Read the model definition and answer for the solid it produces. Units are mm, in the model's axes. A direction names the side the tool comes from. Round coordinates to 2 decimals unless told otherwise and drop trailing zeros. Write each loop counter-clockwise with the first axis right and the second up, starting at its lowest first coordinate (ties: lowest second). Pieces come first, ordered by that corner, then holes. Notation, with made-up numbers: M -29.75,-4.5 L -3.75,-4.5 A20 ccw -3.75,6.5 Z; hole C 80,-27.75 d11. An arc over 180 degrees is marked long. Use one line per item in the form item = value. Start each with the question number.
```python
from build123d import *

# Parameters (mm, degrees)
SKETCH3_W               = 6.6929
SKETCH3_H               = 0.635
CUT_EXTRUDE1_DEPTH      = 10.470513559
CUT_EXTRUDE1_DEPTH_BACK = 10.470513559
FILLET1_R               = 0.803148
FILLET2_R               = 0.5220462
FILLET3_R               = 0.15875


with BuildPart() as part:
    # Sketch3 → Revolve1 (revolve)
    with BuildSketch(Plane(origin=(0, 0, 0), x_dir=(1, 0, 0), z_dir=(0, 1, 0))):
        with Locations((-3.34645, 0)):
            Rectangle(SKETCH3_W, SKETCH3_H)
    revolve(axis=Axis((0, 0, -0.3175), (0, 0, 1)))

    # Sketch4 → Cut-Extrude1 (cut, two sides: drawn at the far end of the back side and taken through both)
    with BuildSketch(Plane.XY.offset(-CUT_EXTRUDE1_DEPTH_BACK)):
        with BuildLine():
            Line((0.719953916, 2.528395058), (1.317615519, 4.62731363))
            ThreePointArc((1.317615519, 4.62731363), (3.839760531, 2.89903107), (4.811251613, 0))
            Line((4.811251613, 0), (2.6289, 0))
            ThreePointArc((2.6289, 0), (2.528395058, -0.719953916), (2.234565, -1.384859008))
            Line((2.234565, -1.384859008), (3.041609986, -5.961838567))
            ThreePointArc((3.041609986, -5.961838567), (0, -6.6929), (-3.041609986, -5.961838567))
            Line((-3.041609986, -5.961838567), (-2.234565, -1.384859008))
            ThreePointArc((-2.234565, -1.384859008), (-2.528395058, -0.719953916), (-2.6289, 0))
            Line((-2.6289, 0), (-4.811251613, 0))
            ThreePointArc((-4.811251613, 0), (-3.839760531, 2.89903107), (-1.317615519, 4.62731363))
            Line((-1.317615519, 4.62731363), (-0.719953916, 2.528395058))
            ThreePointArc((-0.719953916, 2.528395058), (0, 2.6289), (0.719953916, 2.528395058))
        make_face()
    extrude(amount=CUT_EXTRUDE1_DEPTH + CUT_EXTRUDE1_DEPTH_BACK, mode=Mode.SUBTRACT)

    # Fillet1
    fillet1_edges = [part.edges().sort_by_distance(p)[0] for p in [
        (1.317615519, 4.62731363, 0),
        (4.811251613, 0, 0),
        (-4.811251613, 0, 0),
        (-1.317615519, 4.62731363, 0),
    ]]
    fillet(fillet1_edges, radius=FILLET1_R)

    # Fillet2
    fillet2_edges = [part.edges().sort_by_distance(p)[0] for p in [
        (3.041609986, -5.961838567, 0),
        (-3.041609986, -5.961838567, 0),
    ]]
    fillet(fillet2_edges, radius=FILLET2_R)

    # Fillet3
    fillet3_edges = [part.edges().sort_by_distance(p)[0] for p in [
        (-0.719953916, 2.528395058, 0),
        (0.719953916, 2.528395058, 0),
        (2.6289, 0, 0),
        (2.234565, -1.384859008, 0),
        (-2.234565, -1.384859008, 0),
        (-2.6289, 0, 0),
    ]]
    fillet(fillet3_edges, radius=FILLET3_R)


solid = part.part
```
Q1. A tool of negligible diameter and unlimited length cuts with its end or side. For faces 1 (the face through (4.555, 0.303, 0.004)), 2 (the face through (0, 3, 0.318)), from which of +Z, -Z, +X, -X, +Y, -Y can it reach the whole face along a straight path? Write none if from no direction.
Q2. Straight lines are drawn through the part: line 1 (X direction, y = 4.25, z = 0.05); line 2 (X direction, y = 3, z = 0.25); line 3 (X direction, y = -0.5, z = -0.1). For each, find the intervals that lie inside material, in ascending order. Write a range as [from, to].
Q3. Find section C-C on x = 4.5. Write down the section's boundary in (y, z), and give its area (3 significant figures).
Q4. Find section A-A on y = 3. Write down the section's boundary in (x, z).
Q5. For a pull along Y with two mould halves and no side action, classify faces 3 (the face through (0, 3, -0.318)), 4 (the face through (0.24, 6.69, 0)), 5 (the face through (-4.543, 0.288, 0.004)) as +Y half, -Y half, draft (parallel to the pull), parting line (faces both ways), or undercut.
Q6. This flat-tipped pin is pushed along its axis until it touches: pin 1 Ø6 at (x, y) = (0.5, 0) entering from -Z. Where does it stop, or does it pass through?
Q7. Find section D-D on y = -0.75. Write down the section's boundary in (x, z), and give its area (3 significant figures).
Q8. Find section B-B on z = 0.15. Write down the section's boundary in (x, y).
Response:
q1.face_1 = +Z, -Z
q1.face_2 = +Z, +X, -X, +Y, -Y
q2.line_1 = [-5.17, -2.26], [-1.44, 1.44], [2.26, 5.17]
q2.line_2 = [-5.98, -3.76], [-0.85, 0.85], [3.76, 5.98]
q2.line_3 = [-6.67, -2.58], [2.58, 6.67]
q3.outline = M -4.95,-0.32 L 0.24,-0.32 L 0.24,0.32 L -4.95,0.32 Z; M 1.7,-0.32 L 4.95,-0.32 L 4.95,0.32 L 1.7,0.32 Z
q3.area = 5.36 mm²
q4.outline = M -5.98,-0.32 L -3.76,-0.32 L -3.76,0.32 L -5.98,0.32 Z; M -0.85,-0.32 L 0.85,-0.32 L 0.85,0.32 L -0.85,0.32 Z; M 3.76,-0.32 L 5.98,-0.32 L 5.98,0.32 L 3.76,0.32 Z
q5.face_3 = draft
q5.face_4 = parting line
q5.face_5 = undercut
q6.pin_1 = -0.32
q7.outline = M -6.65,-0.32 L -2.52,-0.32 L -2.52,0.32 L -6.65,0.32 Z; M 2.52,-0.32 L 6.65,-0.32 L 6.65,0.32 L 2.52,0.32 Z
q7.area = 5.25 mm²
q8.outline = M -4.71,0.96 A4.81 cw -2.22,4.27 A0.8 cw -1.08,3.78 L -0.76,2.68 A0.16 ccw -0.57,2.57 A2.63 cw 0.57,2.57 A0.16 ccw 0.76,2.68 L 1.08,3.78 A0.8 cw 2.22,4.27 A4.81 cw 4.71,0.96 A0.8 cw 3.93,0 L 2.78,0 A0.16 ccw 2.62,-0.15 A2.63 cw 2.26,-1.34 A0.16 ccw 2.24,-1.44 L 2.91,-5.22 A0.52 ccw 3.72,-5.57 A6.69 ccw long -3.72,-5.57 A0.52 ccw -2.91,-5.22 L -2.24,-1.44 A0.16 ccw -2.26,-1.34 A2.63 cw -2.62,-0.15 A0.16 ccw -2.78,0 L -3.93,0 A0.8 cw Z
